from build123d import *

# Parameters (mm, degrees)
F0_R          = 10.5
F1_DEPTH      = 3
F2_R          = 2
F3_R          = 7
F4_DEPTH      = 0.5
F5_W          = 1.5
F5_H          = 20
F7_R          = 2
F8_DEPTH      = 2.5
F8_DEPTH_BACK = 2.5
F9_T8_DEPTH   = 9.7284161474
F9_T13_DEPTH  = 9.7284161474
F9_T16_ANGLE  = 129.7914851202
F9_T20_DEPTH  = 9.7284161474
F9_T23_ANGLE  = 129.7914851202
F9_T27_DEPTH  = 9.7284161474


# Not quite as in the source:
# - a fillet or chamfer that OpenCascade refuses, or shapes differently, is made with other operations: its cross-section is extruded or revolved along the edge and cut away or added


with BuildPart() as f1:
    # F0 (on Top) → F1 (new body)
    with BuildSketch(Plane.XY):
        Circle(F0_R)
    extrude(amount=F1_DEPTH)

    # F2
    f2_edges = [f1.edges().sort_by_distance(p)[0] for p in [
        (-10.5, 0, 3),
    ]]
    fillet(f2_edges, radius=F2_R)

    # F3 (on face) → F4 (cut)
    with BuildSketch(Plane(origin=(0, 0, 0), x_dir=(1, 0, 0), z_dir=(0, 0, -1))):
        Circle(F3_R)
    extrude(amount=-F4_DEPTH, mode=Mode.SUBTRACT)

    # F5 (on Front) → F6 (revolve)
    with BuildSketch(Plane.XZ):
        with Locations((7.75, -10)):
            Rectangle(F5_W, F5_H)
    revolve(axis=Axis((0, 0, -11.0487695783), (0, 0, -1)))

    # F7 (on Front) → F8 (join, two sides)
    with BuildSketch(Plane.XZ) as f8_sk:
        with BuildLine():
            Line((-5.4332236548, 9.5456002665), (-8.5, 3))
            Line((-8.5, 3), (8.5, 3))
            Line((8.5, 3), (5.4332236548, 9.5456002665))
            ThreePointArc((5.4332236548, 9.5456002665), (0, 13), (-5.4332236548, 9.5456002665))
        make_face()
        with Locations((0, 8)):
            Circle(F7_R, mode=Mode.SUBTRACT)
    extrude(amount=F8_DEPTH)
    extrude(f8_sk.sketch, amount=-F8_DEPTH_BACK)

    # F9: fillet of radius 1 on 4 edges, made by hand

    # F9_s1 → F9_t2 (revolve, cut)
    with BuildSketch(Plane.XY.offset(8)):
        with BuildLine():
            ThreePointArc((3, 2.5), (2.2928932188, 2.2071067812), (2, 1.5))
            Line((2, 1.5), (2, 2.5))
            Line((2, 2.5), (3, 2.5))
        make_face()
    revolve(axis=Axis((0, 2.5, 8), (0, -1, 0)), mode=Mode.SUBTRACT)

    # F9_s3 → F9_t4 (revolve, cut)
    with BuildSketch(Plane.XY.offset(8)):
        with BuildLine():
            ThreePointArc((3, -2.5), (2.2928932188, -2.2071067812), (2, -1.5))
            Line((2, -1.5), (2, -2.5))
            Line((2, -2.5), (3, -2.5))
        make_face()
    revolve(axis=Axis((0, -2.5, 8), (0, -1, 0)), mode=Mode.SUBTRACT)


with BuildPart() as f9_tool6:
    # F9_s7 → F9_t8 (new body)
    with BuildSketch(Plane(origin=(1.4381178705, 0, -3.0694591509), x_dir=(0, 1, 0), z_dir=(-0.4242667111, 0, 0.9055372758))):
        with BuildLine():
            ThreePointArc((-1.5, -8.9698669776), (-2.2071067812, -8.6769737588), (-2.5, -7.9698669776))
            Line((-2.5, -7.9698669776), (-2.5, -8.9698669776))
            Line((-2.5, -8.9698669776), (-1.5, -8.9698669776))
        make_face()
    extrude(amount=F9_T8_DEPTH)

    split(bisect_by=Plane.XY.offset(3), keep=Keep.TOP)


with BuildPart() as f1_1:
    add(f1.part)

    # F9_t5: cut F9_tool6
    add(f9_tool6.part, mode=Mode.SUBTRACT)


with BuildPart() as f9_tool11:
    # F9_s12 → F9_t13 (new body)
    with BuildSketch(Plane(origin=(1.4381178705, 0, -3.0694591509), x_dir=(0, 1, 0), z_dir=(-0.4242667111, 0, 0.9055372758))):
        with BuildLine():
            ThreePointArc((2.5, -7.9698669776), (2.2071067812, -8.6769737588), (1.5, -8.9698669776))
            Line((1.5, -8.9698669776), (2.5, -8.9698669776))
            Line((2.5, -8.9698669776), (2.5, -7.9698669776))
        make_face()
    extrude(amount=F9_T13_DEPTH)

    split(bisect_by=Plane.XY.offset(3), keep=Keep.TOP)


with BuildPart() as f1_2:
    add(f1_1.part)

    # F9_t10: cut F9_tool11
    add(f9_tool11.part, mode=Mode.SUBTRACT)

    # F9_s15 → F9_t16 (revolve, cut)
    with BuildSketch(Plane(origin=(-2.6893252524, 0, 5.7399843051), x_dir=(0, 1, 0), z_dir=(0.4242667111, 0, -0.9055372758))):
        with BuildLine():
            ThreePointArc((2.5, 7.9698669776), (2.2071067812, 8.6769737588), (1.5, 8.9698669776))
            Line((1.5, 8.9698669776), (2.5, 8.9698669776))
            Line((2.5, 8.9698669776), (2.5, 7.9698669776))
        make_face()
    revolve(axis=Axis((0, 2.5, 7), (0, -1, 0)), revolution_arc=F9_T16_ANGLE, mode=Mode.SUBTRACT)


with BuildPart() as f9_tool18:
    # F9_s19 → F9_t20 (new body)
    with BuildSketch(Plane(origin=(2.6893252524, 0, 5.7399843051), x_dir=(0, 1, 0), z_dir=(-0.4242667111, 0, -0.9055372758))):
        with BuildLine():
            ThreePointArc((2.5, -7.9698669776), (2.2071067812, -8.6769737588), (1.5, -8.9698669776))
            Line((1.5, -8.9698669776), (2.5, -8.9698669776))
            Line((2.5, -8.9698669776), (2.5, -7.9698669776))
        make_face()
    extrude(amount=F9_T20_DEPTH)

    split(bisect_by=Plane.XY.offset(3), keep=Keep.TOP)


with BuildPart() as f1_3:
    add(f1_2.part)

    # F9_t17: cut F9_tool18
    add(f9_tool18.part, mode=Mode.SUBTRACT)

    # F9_s22 → F9_t23 (revolve, cut)
    with BuildSketch(Plane(origin=(-2.6893252524, 0, 5.7399843051), x_dir=(0, 1, 0), z_dir=(0.4242667111, 0, -0.9055372758))):
        with BuildLine():
            ThreePointArc((-2.5, 7.9698669776), (-2.2071067812, 8.6769737588), (-1.5, 8.9698669776))
            Line((-1.5, 8.9698669776), (-2.5, 8.9698669776))
            Line((-2.5, 8.9698669776), (-2.5, 7.9698669776))
        make_face()
    revolve(axis=Axis((0, -2.5, 7), (0, -1, 0)), revolution_arc=F9_T23_ANGLE, mode=Mode.SUBTRACT)


with BuildPart() as f9_tool25:
    # F9_s26 → F9_t27 (new body)
    with BuildSketch(Plane(origin=(2.6893252524, 0, 5.7399843051), x_dir=(0, 1, 0), z_dir=(-0.4242667111, 0, -0.9055372758))):
        with BuildLine():
            ThreePointArc((-1.5, -8.9698669776), (-2.2071067812, -8.6769737588), (-2.5, -7.9698669776))
            Line((-2.5, -7.9698669776), (-2.5, -8.9698669776))
            Line((-2.5, -8.9698669776), (-1.5, -8.9698669776))
        make_face()
    extrude(amount=F9_T27_DEPTH)

    split(bisect_by=Plane.XY.offset(3), keep=Keep.TOP)


with BuildPart() as f1_4:
    add(f1_3.part)

    # F9_t24: cut F9_tool25
    add(f9_tool25.part, mode=Mode.SUBTRACT)


solid = f1_4.part
Design review of the part built by this model. Coordinates are the model's own, in mm. A direction names the side the tool comes from. Coordinates: 2 decimals unless noted, no trailing zeros. Loops run counter-clockwise (first coordinate to the right, second up) from the corner with the lowest first, then second, coordinate; pieces in that order, holes last. Notation, with made-up numbers: (-34.75, -25) - (-22.75, -25) arc R6 ccw to (-22.75, -17) - close; hole circle Ø1 at (17, -35.75). An arc over 180 degrees is marked (long way). Use CSV: the item, a comma, the result in double quotes. Start each with the question number.
1. To check wall thickness, follow probe 1 along Z at (x, y) = (0, 0.8); probe 2 along X at (y, z) = (0, -17); probe 3 along Z at (x, y) = (-7.5, -4.25). State the ranges of each line that lie inside material, in increasing order.
2. Add section B-B on z = -6.5. Give the boundary of the cut face in (x, y).
3. Clearance check with flat-ended pins moving along their axes: pin 1 (2.5 mm diameter, centred on x = 2, z = 9.5, fed in from -Y); pin 2 (2.5 mm diameter, centred on x = 2.5, z = 7, fed in from +Y); pin 3 (3 mm diameter, centred on x = -7.5, z = -16.5, fed in from +Y). State where each tip first meets the part, or that it passes through.
4. For faces 4 (the cylindrical face through (-6.687, -2.199, 6.198)), 5 (the flat face through (-0.1, 2.5, 4.6)), 6 (the flat face through (-0.1, -2.5, 4.6)), 7 (the cylindrical face through (6.466, 2.681, -9.606)), 8 (the cylindrical face through (0, 0, 13)), list the 3-axis set-ups (+Z, -Z, +X, -X, +Y, -Y) from which the entire face can be reached by the end or side of a thin tool; tool diameter is ignored.
5. Mouldability with a two-part tool opening along X and no side actions: class faces 1 (the flat face through (-2, -7, -20)), 2 (the cylindrical face through (0, 0, 10)), 3 (the flat face through (-6.945, -0.021, 6.319)) as released by +X, released by -X, zero draft, split by the parting line, or undercut.
6. Add section A-A on x = 0. Give the boundary of the cut face in (y, z).
Resolved:
1,probe 1,"0.5 to 6, 10 to 13"
1,probe 2,"-8.5 to -7, 7 to 8.5"
1,probe 3,"0 to 3"
2,outline,"circle Ø17 at (0, 0); hole circle Ø14 at (0, 0)"
3,pin 1,"y = -2.5"
3,pin 2,"y = 2.5"
3,pin 3,"y = 6.02"
4,face 4,"+Z, -X, -Y"
4,face 5,"+Z, +X, -X, +Y"
4,face 6,"+Z, +X, -X, -Y"
4,face 7,"-Z"
4,face 8,"+Z, +Y, -Y"
5,face 1,"zero draft"
5,face 2,"undercut"
5,face 3,"released by -X"
6,outline,"(-10.5, 0) - (-8.5, 0) - (-8.5, -20) - (-7, -20) - (-7, 0.5) - (7, 0.5) - (7, -20) - (8.5, -20) - (8.5, 0) - (10.5, 0) - (10.5, 1) arc R2 ccw to (8.5, 3) - (2.5, 3) - (2.5, 5) arc R1 ccw to (1.5, 6) - (-1.5, 6) arc R1 ccw to (-2.5, 5) - (-2.5, 3) - (-8.5, 3) arc R2 ccw to (-10.5, 1) - close; (-2.5, 11) arc R1 ccw to (-1.5, 10) - (1.5, 10) arc R1 ccw to (2.5, 11) - (2.5, 12) arc R1 ccw to (1.5, 13) - (-1.5, 13) arc R1 ccw to (-2.5, 12) - close"
